from build123d import *

# Parameters (mm, degrees)
SKETCH1_W           = 60
SKETCH1_H           = 47
BOSS_EXTRUDE1_DEPTH = 2
SKETCH2_W           = 40
SKETCH2_H           = 11
CUT_EXTRUDE1_DEPTH  = 2
CUT_EXTRUDE2_DEPTH  = 2
CUT_EXTRUDE3_DEPTH  = 2
CUT_EXTRUDE4_DEPTH  = 2
CUT_EXTRUDE5_DEPTH  = 2
FILLET1_R           = 2


with BuildPart() as part:
    # Sketch1 → Boss-Extrude1 (new body)
    with BuildSketch(Plane.XY):
        Rectangle(SKETCH1_W, SKETCH1_H)
    extrude(amount=BOSS_EXTRUDE1_DEPTH)

    # Sketch2 → Cut-Extrude1 (cut)
    with BuildSketch(Plane(origin=(0, 0, 0), x_dir=(-1, 0, 0), z_dir=(0, 0, -1))):
        with Locations((0, -18)):
            Rectangle(SKETCH2_W, SKETCH2_H)
    extrude(amount=-CUT_EXTRUDE1_DEPTH, mode=Mode.SUBTRACT)

    # Sketch3 → Cut-Extrude2 (cut)
    with BuildSketch(Plane(origin=(0, 0, 0), x_dir=(-1, 0, 0), z_dir=(0, 0, -1))):
        with BuildLine():
            Line((27, -13), (27, -19))
            ThreePointArc((27, -19), (25, -21), (23, -19))
            Line((23, -19), (23, -13))
            ThreePointArc((23, -13), (25, -11), (27, -13))
        make_face()
    cut_extrude2 = extrude(amount=-CUT_EXTRUDE2_DEPTH, mode=Mode.SUBTRACT)

    # Sketch4 → Cut-Extrude3 (cut)
    with BuildSketch(Plane(origin=(0, 0, 0), x_dir=(-1, 0, 0), z_dir=(0, 0, -1))):
        with BuildLine():
            Line((27, 19), (27, 13))
            ThreePointArc((27, 13), (25, 11), (23, 13))
            Line((23, 13), (23, 19))
            ThreePointArc((23, 19), (25, 21), (27, 19))
        make_face()
    cut_extrude3 = extrude(amount=-CUT_EXTRUDE3_DEPTH, mode=Mode.SUBTRACT)

    # Sketch5 → Cut-Extrude4 (cut)
    with BuildSketch(Plane(origin=(0, 0, 0), x_dir=(-1, 0, 0), z_dir=(0, 0, -1))):
        with BuildLine():
            Line((12.5, -5.5), (18.5, -5.5))
            ThreePointArc((18.5, -5.5), (20, -7), (18.5, -8.5))
            Line((18.5, -8.5), (12.5, -8.5))
            ThreePointArc((12.5, -8.5), (11, -7), (12.5, -5.5))
        make_face()
    cut_extrude4 = extrude(amount=-CUT_EXTRUDE4_DEPTH, mode=Mode.SUBTRACT)

    # Sketch6 → Cut-Extrude5 (cut)
    with BuildSketch(Plane(origin=(0, 0, 0), x_dir=(-1, 0, 0), z_dir=(0, 0, -1))):
        with BuildLine():
            Line((12.5, 5.5), (18.5, 5.5))
            ThreePointArc((18.5, 5.5), (20, 4), (18.5, 2.5))
            Line((18.5, 2.5), (12.5, 2.5))
            ThreePointArc((12.5, 2.5), (11, 4), (12.5, 5.5))
        make_face()
    cut_extrude5 = extrude(amount=-CUT_EXTRUDE5_DEPTH, mode=Mode.SUBTRACT)

    # Mirror1: Cut-Extrude2, Cut-Extrude3, Cut-Extrude4, Cut-Extrude5 across plane
    add(cut_extrude2.mirror(Plane.ZY), mode=Mode.SUBTRACT)
    add(cut_extrude3.mirror(Plane.ZY), mode=Mode.SUBTRACT)
    add(cut_extrude4.mirror(Plane.ZY), mode=Mode.SUBTRACT)
    add(cut_extrude5.mirror(Plane.ZY), mode=Mode.SUBTRACT)

    # Fillet1
    fillet1_edges = [part.edges().sort_by_distance(p)[0] for p in [
        (-20, -12.5, 1),
        (-20, -23.5, 1),
        (20, -23.5, 1),
        (20, -12.5, 1),
        (30, -23.5, 1),
        (-30, -23.5, 1),
        (-30, 23.5, 1),
        (30, 23.5, 1),
    ]]
    fillet(fillet1_edges, radius=FILLET1_R)


solid = part.part
Geometry check sheet. Reference: the model listing, model coordinates, mm. A direction names the side the tool comes from. Round coordinates to 2 decimals unless told otherwise and drop trailing zeros. Write each loop counter-clockwise with the first axis right and the second up, starting at its lowest first coordinate (ties: lowest second). Pieces come first, ordered by that corner, then holes.
Item 1: Section check A-A (y = -7). Record the boundary of the cut face in (x, z).
Determined:
outline: (-30, 0) - (-20, 0) - (-20, 2) - (-30, 2) - close; (-11, 0) - (11, 0) - (11, 2) - (-11, 2) - close; (20, 0) - (30, 0) - (30, 2) - (20, 2) - close
Item 2: Section check C-C (y = -16). Record the boundary of the cut face in (x, z).
Determined:
outline: (-30, 0) - (-27, 0) - (-27, 2) - (-30, 2) - close; (-23, 0) - (-20, 0) - (-20, 2) - (-23, 2) - close; (20, 0) - (23, 0) - (23, 2) - (20, 2) - close; (27, 0) - (30, 0) - (30, 2) - (27, 2) - close
Item 3: Section check B-B (x = 14.5). Record the boundary of the cut face in (y, z), plus the area to 3 significant figures.
Determined:
outline: (-12.5, 0) - (-8.5, 0) - (-8.5, 2) - (-12.5, 2) - close; (-5.5, 0) - (2.5, 0) - (2.5, 2) - (-5.5, 2) - close; (5.5, 0) - (23.5, 0) - (23.5, 2) - (5.5, 2) - close
area: 60.0 mm2
Item 4: Go/stop test with a flat-tipped pin: pin 1 Ø6 at (x, y) = (6, -5.5) entering from -Z. Record where the tip stops, or that it passes through.
Determined:
pin 1: stops at z = 0
Item 5: Material ranges on line 1 along X through (y, z) = (4, 1.2); line 2 along X through (y, z) = (18, 1.8); line 3 along X through (y, z) = (-17, 1.55), recorded low to high.
Determined:
line 1: x = -30 to -20, -11 to 11, 20 to 30
line 2: x = -30 to -27, -23 to 23, 27 to 30
line 3: x = -30 to -27, -23 to -20, 20 to 23, 27 to 30
Item 6: Section check D-D (x = -1). Record the boundary of the cut face in (y, z).
Determined:
outline: (-12.5, 0) - (23.5, 0) - (23.5, 2) - (-12.5, 2) - close
Item 7: Mould release check, pull along Y, two halves, no side actions. Record for faces 4 (the face through (-30, 0, 1)), 5 (the face through (-25, -11, 1)), 6 (the face through (25, -23.5, 1)), 7 (the face through (25, 11, 1)): +Y half, -Y half, draft (parallel to the pull), parting line (faces both ways), or undercut.
Determined:
face 4: draft
face 5: undercut
face 6: -Y half
face 7: undercut
Item 8: Access from +Z, -Z, +X, -X, +Y, -Y to the whole of each face (thin tool, end or side, straight path). Record for faces 1 (the face through (-25, -23.5, 1)), 2 (the face through (20.6, -22.93, 1.01)), 3 (the face through (-23, -16, 1)).
Determined:
face 1: +Z, -Z, +X, -X, -Y
face 2: +Z, -Z, -Y
face 3: +Z, -Z
